```python
from build123d import *

# Parameters (mm, degrees)
F1_DEPTH = 63.5
F2_DEPTH = 25.4
F3_DEPTH = 6.35


with BuildPart() as f1:
    # F0 (on Front) → F1 (new body, symmetric)
    with BuildSketch(Plane.XZ):
        Polygon((-31.75, -19.05), (31.75, -19.05), (31.75, 19.05), (6.35, 19.05), (-31.75, 19.05), align=None)
    extrude(amount=F1_DEPTH, both=True)

    # F0 (on Front) → F2 (join, symmetric)
    with BuildSketch(Plane.XZ):
        with BuildLine():
            Line((6.35, 19.05), (31.75, 19.05))
            Line((31.75, 19.05), (31.75, 43.1967032691))
            ThreePointArc((31.75, 43.1967032691), (40.3541311515, 63.9689133875), (61.1263412699, 72.573044539))
            Line((61.1263412699, 72.573044539), (78.5394700097, 72.573044539))
            Line((78.5394700097, 72.573044539), (78.5394700097, 97.973044539))
            Line((78.5394700097, 97.973044539), (61.1263412699, 97.973044539))
            ThreePointArc((61.1263412699, 97.973044539), (22.3936189094, 81.9294256296), (6.35, 43.1967032691))
            Line((6.35, 43.1967032691), (6.35, 19.05))
        make_face()
        Polygon((111.9425526827, 97.973044539), (78.5394700097, 97.973044539), (78.5394700097, 72.573044539), (111.903113532, 72.573044539), align=None)
    extrude(amount=F2_DEPTH, both=True)

    # F0 (on Front) → F3 (join, symmetric)
    with BuildSketch(Plane.XZ):
        with BuildLine():
            add(Edge.make_bspline(
                [(-31.75, 19.05), (-33.8824763894, 62.8609061241), (23.62857759, 116.8053820729), (78.5394700097, 97.973044539)],
                knots=[0, 0, 0, 0, 135.6193723415, 135.6193723415, 135.6193723415, 135.6193723415], degree=3))
            Line((-31.75, 19.05), (6.35, 19.05))
            Line((6.35, 19.05), (6.35, 43.1967032691))
            ThreePointArc((6.35, 43.1967032691), (22.3936189094, 81.9294256296), (61.1263412699, 97.973044539))
            Line((61.1263412699, 97.973044539), (78.5394700097, 97.973044539))
        make_face()
    extrude(amount=F3_DEPTH, both=True)

    # F0 (on Front) → F4 (revolve)
    with BuildSketch(Plane.XZ):
        Polygon((111.9605090454, 109.5374825459), (111.9425526827, 97.973044539), (111.903113532, 72.573044539), (111.9013503194, 71.4374825459), (134.4194700097, 71.4374825459), (134.4194700097, 109.5374825459), align=None)
    revolve(axis=Axis((111.9309296824, 0, 90.4874825459), (0.0015527206, 0, 0.9999987945)))


solid = f1.part
```
CAD build for the part. Positions are in the model's coordinates, mm. A direction names the side the tool comes from. Coordinates: 2 decimals unless noted, no trailing zeros. Write each loop counter-clockwise with the first axis right and the second up, starting at its lowest first coordinate (ties: lowest second). Pieces come first, ordered by that corner, then holes. Notation, with made-up numbers: (83, 38.25) -> (95, 38.25) arc R4 cw to (95, 43.25) -> close; hole circle Ø2 at (56, 28.5). An arc over 180 degrees is marked (long way). Return JSON: item names as keys, results as strings. Group by question number.
Q1. Drill centre lines: line 1 (Z direction, x = 110.5, y = -17); line 2 (X direction, y = 8.5, z = 29); line 3 (Z direction, x = -20, y = 20). Where is each one in solid material? Low to high.
Q2. Flat gauge pins, fed straight in: pin 1 (5.5 mm diameter, centred on y = 18, z = 32, fed in from -X); pin 2 (11.5 mm diameter, centred on y = 1.5, z = 3.5, fed in from -X); pin 3 (4 mm diameter, centred on y = -32.5, z = 4, fed in from +X). Where does each tip first touch, or does it go through?
Q3. Cut at A-A, the plane y = 31.5. Give the cut face in (x, z).
Q4. Which spindle directions (+Z, -Z, +X, -X, +Y, -Y) get a long thin tool onto all of the face, cutting with end or side? Do faces 1 (the face through (22.82, 15.74, 82.35)), 2 (the face through (40.13, -0.36, 63.74)). Say none if no direction does.
Returned:
{
 "1": {"line 1": "z = 71.47 to 109.57", "line 2": "x = 6.35 to 31.75", "line 3": "z = -19.05 to 19.05"},
 "2": {"pin 1": "stops at x = 6.35", "pin 2": "stops at x = -31.75", "pin 3": "stops at x = 31.75"},
 "3": {"outline": "(-31.75, -19.05) -> (31.75, -19.05) -> (31.75, 19.05) -> (-31.75, 19.05) -> close"},
 "4": {"face 1": "+Z, -X, +Y", "face 2": "-Z, +Y, -Y"}
}
